Geometry check sheet. Reference: drawing and pictorial views, mm from the part's lowest x, y, z. A direction names the side the tool comes from. Give positions to 0.01 mm unless a question says otherwise; leave off trailing zeros. Write each loop counter-clockwise with the first axis right and the second up, starting at its lowest first coordinate (ties: lowest second). Pieces come first, ordered by that corner, then holes. Notation, with made-up numbers: M -31.5,-18.5 L -8.5,-18.5 A24 ccw -8.5,15.5 Z; hole C 3.25,26.25 d5. An arc over 180 degrees is marked long. One line per item, written item: value. Start each with the question number.
1. Cross-section at A-A on x = 50.8. Record the cut outline in (y, z) (3 decimals), then the cut area to 3 significant figures.
2. Cross-section at B-B on y = 15. Record the cut outline in (x, z) (3 decimals).
3. Tool access check on the marked faces 1 and 2. Record the directions out of +Z, -Z, +X, -X, +Y, -Y that give a thin tool (end or side, any length) a straight path to the whole face; none if there is none.
4. Scan lines: line 1 (Z direction, x = 50.8, y = 38) (3 decimals); line 2 (X direction, y = 22, z = 38); line 3 (Z direction, x = 136.5, y = 13). Record each from-to range of solid material in increasing order.
5. Gauge pin test, flat ends, axial feed: pin 1 (1 mm diameter, centred on x = 128, y = 15, fed in from +Z); pin 2 (8 mm diameter, centred on x = 163, z = 58.5, fed in from -Y); pin 3 (16.5 mm diameter, centred on y = 11, z = 57, fed in from +X). Record the tip position at first contact, or that the pin passes through.
6. Cross-section at C-C on x = 173.5. Record the cut outline in (y, z), then the cut area to 3 significant figures.
7. Cross-section at D-D on z = 64. Record the cut outline in (x, y), then the cut area to 3 significant figures.
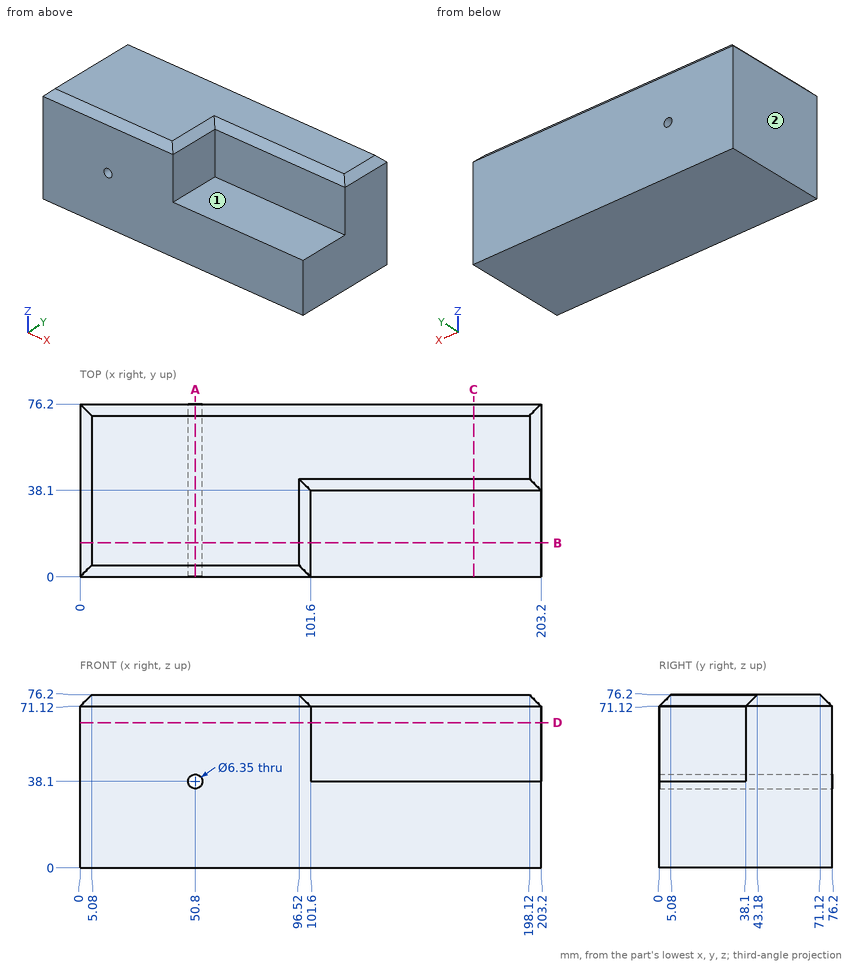
Report:
1. outline: M 0,0 L 76.2,0 L 76.2,34.925 L 0,34.925 Z; M 0,41.275 L 76.2,41.275 L 76.2,71.12 L 71.12,76.2 L 5.08,76.2 L 0,71.12 Z
1. area: 5,300 mm^2
2. outline: M 0,0 L 203.2,0 L 203.2,38.1 L 101.6,38.1 L 101.6,71.12 L 96.52,76.2 L 5.08,76.2 L 0,71.12 Z; hole C 50.8,38.1 d6.35
3. face 1: +Z, +X, -Y
3. face 2: +Z, -Z, -X, +Y, -Y
4. line 1: z = 0 to 34.925, 41.275 to 76.2
4. line 2: x = 0 to 47.63, 53.97 to 203.2
4. line 3: z = 0 to 38.1
5. pin 1: stops at z = 38.1
5. pin 2: stops at y = 38.1
5. pin 3: stops at x = 101.6
6. outline: M 0,0 L 76.2,0 L 76.2,71.12 L 71.12,76.2 L 43.18,76.2 L 38.1,71.12 L 38.1,38.1 L 0,38.1 Z
6. area: 4,330 mm^2
7. outline: M 0,0 L 101.6,0 L 101.6,38.1 L 203.2,38.1 L 203.2,76.2 L 0,76.2 Z
7. area: 11,600 mm^2
